```python
from build123d import *

# Parameters (mm, degrees)
F0_W     = 21.598608559
F0_H     = 10
F0_W_2   = 6.802782882
F0_W_3   = 3.8192358334
F0_H_2   = 5.3111389279
F1_DEPTH = 4.1
F2_DEPTH = 15
F3_W     = 3.9702160284
F3_H     = 3.7578037009
F4_DEPTH = 1.4917735243
F5_R     = 1.3059385841
F6_DEPTH = 10.001
F7_W     = 9.4027826563
F7_H     = 12.5999997742
F7_W_2   = 6.802782882
F7_H_2   = 10
F7_W_3   = 3.8192358334
F7_H_3   = 5.3111389279
F8_DEPTH = 3
F9_R     = 1


with BuildPart() as f1:
    # F0 (on Top) → F1 (new body)
    with BuildSketch(Plane.XY):
        with Locations((-14.2006957205, 0)):
            Rectangle(F0_W, F0_H)
        with Locations((14.2006957205, 0)):
            Rectangle(F0_W, F0_H)
        Rectangle(F0_W_2, F0_H)
        Rectangle(F0_W_3, F0_H_2, mode=Mode.SUBTRACT)
        Rectangle(F0_W_3, F0_H_2)
    extrude(amount=F1_DEPTH)

    # F0 (on Top) → F2 (join)
    with BuildSketch(Plane.XY):
        Rectangle(F0_W_2, F0_H)
        Rectangle(F0_W_3, F0_H_2, mode=Mode.SUBTRACT)
    extrude(amount=F2_DEPTH)

    # F3 (on face) → F4 (cut, through all)
    with BuildSketch(Plane.YZ.offset(3.401391441)):
        with Locations((0, 7.8942701221)):
            Rectangle(F3_W, F3_H)
    extrude(amount=-F4_DEPTH, mode=Mode.SUBTRACT)

    # F5 (on face) → F6 (cut, through all)
    with BuildSketch(Plane.XZ.offset(5)):
        with Locations((-22.0196954906, 2.05)):
            Circle(F5_R)
        with Locations((21.1608465761, 2.05)):
            Circle(F5_R)
    extrude(amount=-F6_DEPTH, mode=Mode.SUBTRACT)

    # F7 (on face) → F8 (join)
    with BuildSketch(Plane.XY.offset(15)):
        Rectangle(F7_W, F7_H)
        Rectangle(F7_W_2, F7_H_2, mode=Mode.SUBTRACT)
        Rectangle(F7_W_2, F7_H_2)
        Rectangle(F7_W_3, F7_H_3, mode=Mode.SUBTRACT)
    extrude(amount=-F8_DEPTH)

    # F9
    f9_edges = [f1.edges().sort_by_distance(p)[0] for p in [
        (-4.701391, 0, 15),
        (0, -6.3, 15),
        (0, -6.3, 12),
        (4.701391, 0, 12),
        (0, 6.3, 15),
        (-4.701391, 0, 12),
        (0, 6.3, 12),
        (4.701391, 0, 15),
        (4.701391, -6.3, 13.5),
        (4.701391, 6.3, 13.5),
        (-4.701391, 6.3, 13.5),
        (-4.701391, -6.3, 13.5),
    ]]
    fillet(f9_edges, radius=F9_R)


solid = f1.part
```
Design review of the part built by this model. Coordinates are the model's own, in mm. A direction names the side the tool comes from. Round coordinates to 2 decimals unless told otherwise and drop trailing zeros. Order: outer loops, then holes, each group sorted by start corner. A loop starts at its lowest first (then second) coordinate and runs counter-clockwise, first axis right, second up. Notation, with made-up numbers: (9.5, -0.5) - (56.5, -0.5) arc R5 cw to (56.5, 6.5) - close; hole circle Ø10 at (-10.5, 58). An arc over 180 degrees is marked (long way). One line per question, with ' | ' between items.
Item 1: Take a section at C-C, the plane x = 21.5. Write out the cut boundary in (y, z), then the cut area to 3 significant figures.
Checks:
outline: (-5, 0) - (5, 0) - (5, 0.79) - (-5, 0.79) - close; (-5, 3.31) - (5, 3.31) - (5, 4.1) - (-5, 4.1) - close | area: 15.8 mm²
Item 2: Machinability: for faces 4 (the face through (3, -1.985, 8)), 5 (the face through (4.401, 0.074, 12.285)), 6 (the face through (-0.1, -6.3, 13.5)), 7 (the face through (1.91, 0, 11)), which of the approach directions +Z, -Z, +X, -X, +Y, -Y give a long, thin tool a straight path to every point of the face, cutting with its end or side? Answer none if there is none.
Checks:
face 4: +X | face 5: +X, +Y, -Y | face 6: +Z, -Z, +X, -X, -Y | face 7: +Z
Item 3: Take a section at A-A, the plane y = -1.25. Write out the cut boundary in (x, z), then the cut area to 3 significant figures.
Checks:
outline: (-25, 0) - (25, 0) - (25, 4.1) - (3.4, 4.1) - (3.4, 6.02) - (1.91, 6.02) - (1.91, 4.1) - (-1.91, 4.1) - (-1.91, 15) - (-3.7, 15) arc R1 ccw to (-4.7, 14) - (-4.7, 13) arc R1 ccw to (-3.7, 12) - (-3.4, 12) - (-3.4, 4.1) - (-25, 4.1) - close; (1.91, 9.77) - (3.4, 9.77) - (3.4, 12) - (3.7, 12) arc R1 ccw to (4.7, 13) - (4.7, 14) arc R1 ccw to (3.7, 15) - (1.91, 15) - close; hole circle Ø2.61 at (-22.02, 2.05); hole circle Ø2.61 at (21.16, 2.05) | area: 228 mm²
Item 4: Take a section at B-B, the plane z = 2.05. Write out the cut boundary in (x, y).
Checks:
outline: (-25, -5) - (-23.33, -5) - (-23.33, 5) - (-25, 5) - close; (-20.71, -5) - (19.85, -5) - (19.85, 5) - (-20.71, 5) - close; (22.47, -5) - (25, -5) - (25, 5) - (22.47, 5) - close
Item 5: Draft analysis for pull direction Y (two halves, no side actions). For faces 1 (the face through (0, 5, 3)), 2 (the face through (3, 0, 6.015)), 3 (the face through (4.701, -0.1, 13.5)), state which applies: +Y half, -Y half, draft (parallel to the pull), parting line (faces both ways), or undercut.
Checks:
face 1: +Y half | face 2: undercut | face 3: draft
Item 6: Wall thickness on line 1 (X direction, y = 3.75, z = 2); line 2 (X direction, y = -1.5, z = 5.75); line 3 (Y direction, x = 1, z = 13.5): over which ranges is each line inside the solid? List them lowest first. Write a range as [from, to].
Checks:
line 1: [-25, -23.32], [-20.71, 19.86], [22.47, 25] | line 2: [-3.4, -1.91], [1.91, 3.4] | line 3: [-6.3, -2.66], [2.66, 6.3]
Item 7: Take a section at D-D, the plane z = 8. Write out the cut boundary in (x, y), then the cut area to 3 significant figures.
Checks:
outline: (-3.4, -5) - (3.4, -5) - (3.4, -1.99) - (1.91, -1.99) - (1.91, -2.66) - (-1.91, -2.66) - (-1.91, 2.66) - (1.91, 2.66) - (1.91, 1.99) - (3.4, 1.99) - (3.4, 5) - (-3.4, 5) - close | area: 41.8 mm²
Item 8: For P1, Ø6.5, axis at y = 0.5, z = 7.5, coming from the -X side; P2, Ø4, axis at y = -0.5, z = 6.5, coming from the +X side; P3, Ø1.6, axis at x = 3, z = 7.5, coming from the -Y side, all flat-tipped, find the tip position at first contact; note any pin that passes through.
Checks:
P1: x = -3.4 | P2: x = 3.4 | P3: y = -5
